Job drawing, mm, ordinate dimensions from the low corner. One solid piece. Coordinates: 2 decimals unless noted, no trailing zeros. Write each loop counter-clockwise with the first axis right and the second up, starting at its lowest first coordinate (ties: lowest second). Pieces come first, ordered by that corner, then holes. Notation, with made-up numbers: (6.25, 31) - (14.25, 31) arc R28 cw to (14.25, 58) - close; hole circle Ø10 at (-23.5, -32.75). An arc over 180 degrees is marked (long way). Put each result on its own line as item: value. Start each with the question number.
1. Saw through at A-A, the plane z = 16. Write the cut outline in (x, y).
2. Saw through at B-B, the plane y = 2.5. Write the cut outline in (x, z) (3 decimals), plus the area to 3 significant figures.
3. Saw through at D-D, the plane x = 26. Write the cut outline in (y, z).
4. Saw through at C-C, the plane x = 107.5. Write the cut outline in (y, z), plus the area to 3 significant figures.
5. Drill centre lines: L1, parallel to X at y = 3.5, z = 30; L2, parallel to Z at x = 84, y = 3; L3, parallel to X at y = 4.5, z = 70. Where is each one in solid material? Low to high. Write a range as from..to.
6. Drop flat-ended pins along their axis: P1, Ø2, axis at x = 85, z = 103, coming from the -Y side; P2, Ø3.5, axis at x = 74.676, z = 61.976, coming from the -Y side; P3, Ø1, axis at x = 15, y = 1, coming from the -Z side. Give the stop position or say it passes through.
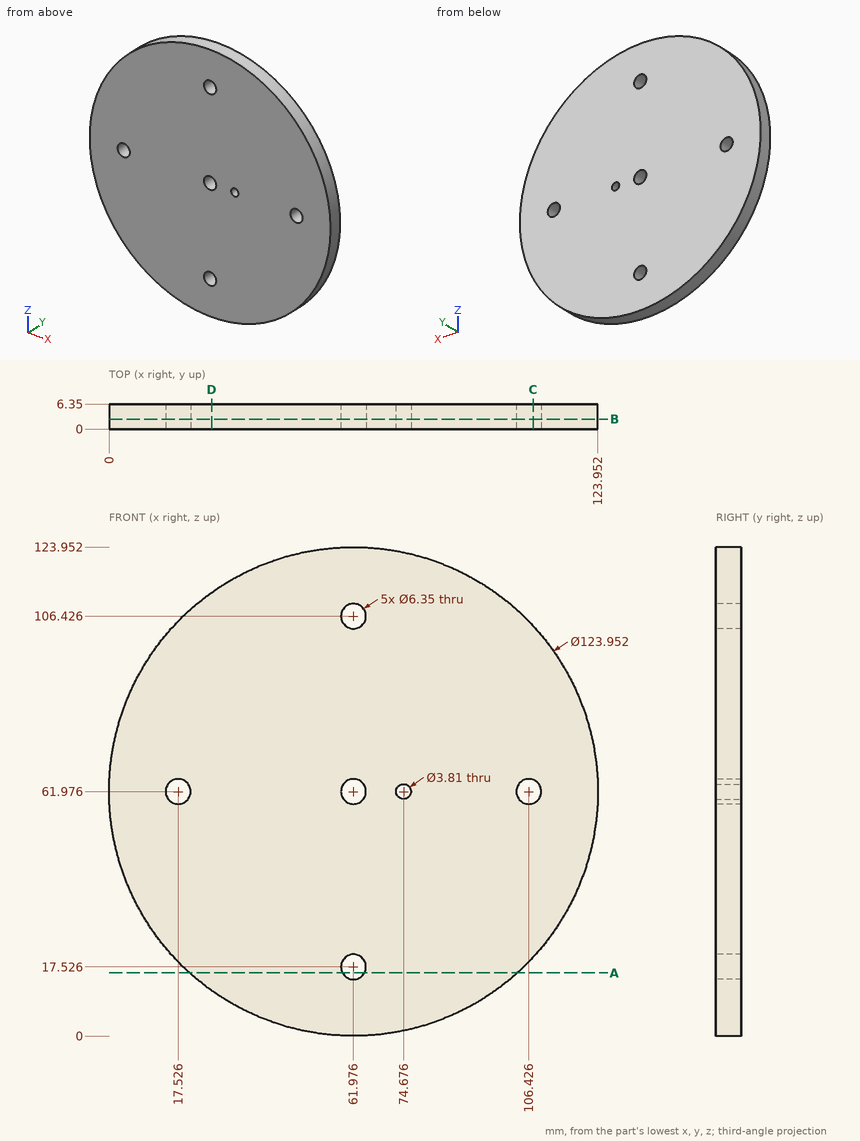
Final values:
1. outline: (20.42, 0) - (59.19, 0) - (59.19, 6.35) - (20.42, 6.35) - close; (64.76, 0) - (103.54, 0) - (103.54, 6.35) - (64.76, 6.35) - close
2. outline: circle Ø123.952 at (61.976, 61.976); hole circle Ø6.35 at (17.526, 61.976); hole circle Ø6.35 at (61.976, 17.526); hole circle Ø6.35 at (61.976, 61.976); hole circle Ø6.35 at (61.976, 106.426); hole circle Ø3.81 at (74.676, 61.976); hole circle Ø6.35 at (106.426, 61.976)
2. area: 11,900 mm²
3. outline: (0, 11.51) - (6.35, 11.51) - (6.35, 112.44) - (0, 112.44) - close
4. outline: (0, 19.92) - (6.35, 19.92) - (6.35, 58.99) - (0, 58.99) - close; (0, 64.96) - (6.35, 64.96) - (6.35, 104.03) - (0, 104.03) - close
4. area: 496 mm²
5. L1: x = 8.89..115.07
5. L2: z = 4.05..119.91
5. L3: x = 0.52..123.43
6. P1: stops at y = 0
6. P2: passes through
6. P3: stops at z = 20.98
